CAD build for the part. Positions are in the model's coordinates, mm. Face numbers are marked on the shaded views. A direction names the side the tool comes from. Round coordinates to 2 decimals unless told otherwise and drop trailing zeros. Write each loop counter-clockwise with the first axis right and the second up, starting at its lowest first coordinate (ties: lowest second). Pieces come first, ordered by that corner, then holes. Notation, with made-up numbers: (12.25, 32) - (41.25, 32) arc R22 cw to (41.25, 59) - close; hole circle Ø8 at (39, 20.25). An arc over 180 degrees is marked (long way). Put each result on its own line as item: value. Start each with the question number.
Item 1: Cut at A-A (x = 0). Give the cut face in (y, z) (1 decimal).
Item 2: Cut at B-B (z = 0). Give the cut face in (x, y) (1 decimal), and give its area (3 significant figures).
Item 3: Drill centre lines: line 1 (Z direction, x = 0, y = 0.25); line 2 (X direction, y = 1.75, z = 0); line 3 (Y direction, x = 6.75, z = 9). Where is each one in solid material? Low to high. Write a range as from..to.
Item 4: Pin check, flat tips, straight feed: pin 1 Ø5 at (x, z) = (7.5, 9.5) entering from +Y; pin 2 Ø2.5 at (x, z) = (7, 9) entering from -Y; pin 3 Ø2 at (y, z) = (-0.5, 3.5) entering from +X. Stop position of each tip, or through.
Item 5: Cut at D-D (x = 5.25). Give the cut face in (y, z), and give its area (3 significant figures).
Item 6: Mould opens along X. For the marked faces 6, 7 and 8 say: released by +X, released by -X, zero draft, split by the parting line, or undercut.
Item 7: Cut at C-C (y = 0.5). Give the cut face in (x, z) (1 decimal).
Item 8: 3-axis set-ups, long thin cutter, end or side, ignore diameter. For the marked faces 1, 2, 3, 4 and 5: which of +Z, -Z, +X, -X, +Y, -Y reach the whole face in a straight line?
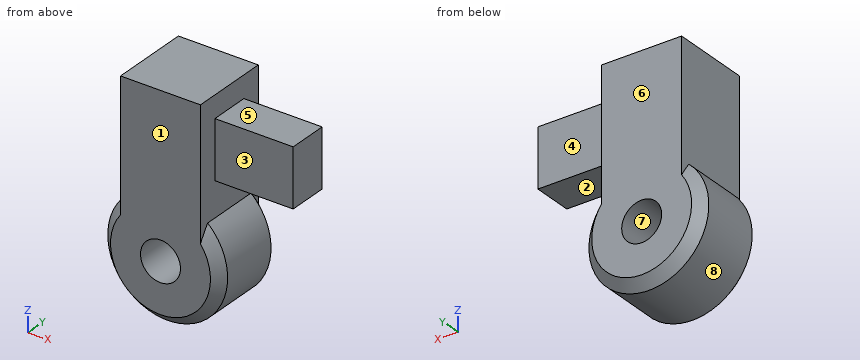
```python
from build123d import *

# Parameters (mm, degrees)
F0_R     = 4.7625
F0_R_2   = 1.5875
F4_DEPTH = 3.175
F1_W     = 6.35
F1_H     = 12.7
F5_DEPTH = 3.175
F3_R     = 1.5875
F6_DEPTH = 12.7
F7_SIZE  = 0.79375
F2_W     = 7.2895279154
F2_H     = 4.6182582155
F8_DEPTH = 1.5875


with BuildPart() as f4:
    # F0 (on Front) → F4 (new body, symmetric)
    with BuildSketch(Plane.XZ):
        Circle(F0_R)
        Circle(F0_R_2, mode=Mode.SUBTRACT)
    extrude(amount=F4_DEPTH, both=True)

    # F1 (on Front) → F5 (join, symmetric)
    with BuildSketch(Plane.XZ):
        with Locations((0, 6.35)):
            Rectangle(F1_W, F1_H)
    extrude(amount=F5_DEPTH, both=True)

    # F3 (on Front) → F6 (cut, symmetric)
    with BuildSketch(Plane.XZ):
        Circle(F3_R)
    extrude(amount=F6_DEPTH, both=True, mode=Mode.SUBTRACT)

    # F7
    f7_edges = [f4.edges().sort_by_distance(p)[0] for p in [
        (0, 3.175, -4.7625),
        (0, -3.175, -4.7625),
    ]]
    chamfer(f7_edges, length=F7_SIZE)

    # F2 (on Front) → F8 (join, symmetric)
    with BuildSketch(Plane.XZ):
        with Locations((5.749846343, 8.6307809688)):
            Rectangle(F2_W, F2_H)
    extrude(amount=F8_DEPTH, both=True)


solid = f4.part
```
Output values:
1. outline: (-3.2, -4) - (-2.4, -4.8) - (2.4, -4.8) - (3.2, -4) - (3.2, -1.6) - (-3.2, -1.6) - close; (-3.2, 1.6) - (3.2, 1.6) - (3.2, 12.7) - (-3.2, 12.7) - close
2. outline: (-4.8, -2.4) - (-4, -3.2) - (-1.6, -3.2) - (-1.6, 3.2) - (-4, 3.2) - (-4.8, 2.4) - close; (1.6, -3.2) - (4, -3.2) - (4.8, -2.4) - (4.8, 2.4) - (4, 3.2) - (1.6, 3.2) - close
2. area: 39.1 mm2
3. line 1: -4.76..-1.59, 1.59..12.7
3. line 2: -4.76..-1.59, 1.59..4.76
3. line 3: -1.59..1.59
4. pin 1: y = 1.59
4. pin 2: y = -1.59
4. pin 3: x = 4.05
5. outline: (-1.59, 6.32) - (1.59, 6.32) - (1.59, 10.94) - (-1.59, 10.94) - close
5. area: 14.7 mm2
6. face 6: zero draft
6. face 7: undercut
6. face 8: split by the parting line
7. outline: (-3.2, 3.5) arc R4.8 ccw (long way) to (3.2, 3.5) - (3.2, 6.3) - (9.4, 6.3) - (9.4, 10.9) - (3.2, 10.9) - (3.2, 12.7) - (-3.2, 12.7) - close; hole circle Ø3.2 at (0, 0)
8. face 1: +Z, -Z, +X, -X, -Y
8. face 2: +X, +Y, -Y
8. face 3: +Z, +X, -Y
8. face 4: +Z, +X, +Y
8. face 5: +Z, +X, +Y, -Y
